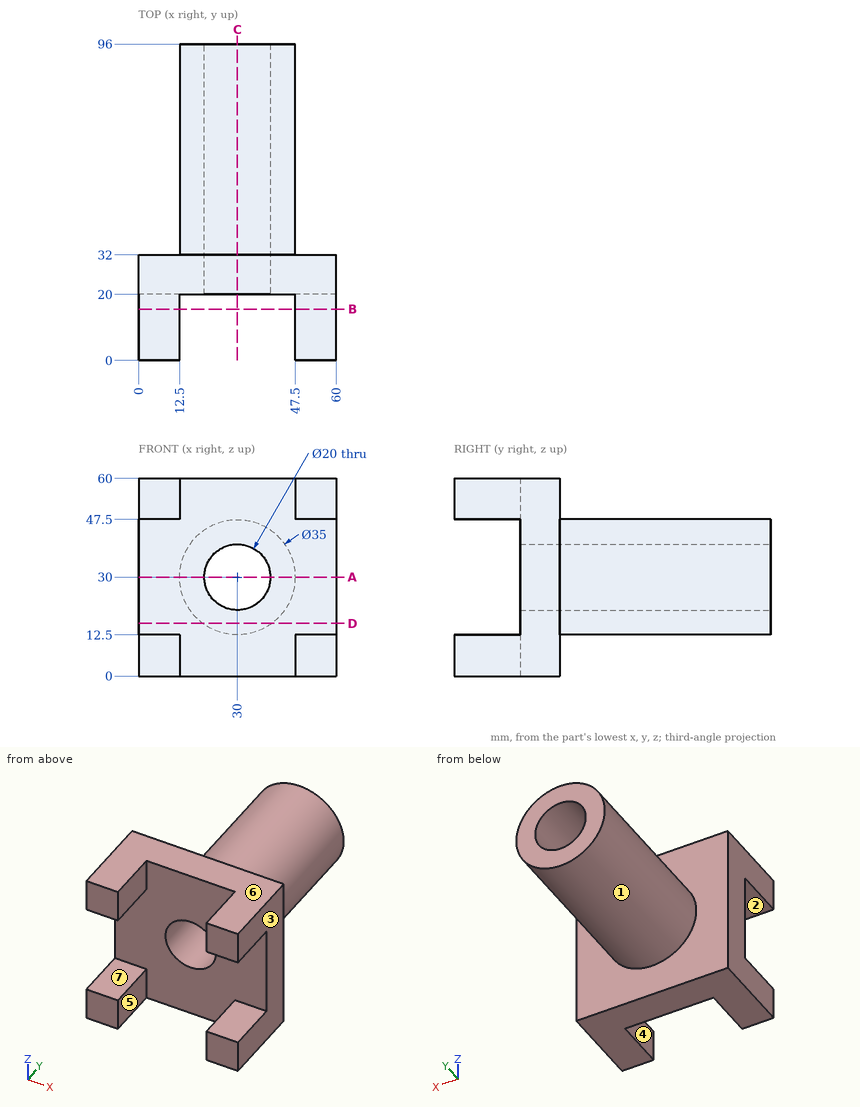
Geometry check sheet. Reference: drawing and pictorial views, mm from the part's lowest x, y, z. A direction names the side the tool comes from. Coordinates: 2 decimals unless noted, no trailing zeros. Write each loop counter-clockwise with the first axis right and the second up, starting at its lowest first coordinate (ties: lowest second). Pieces come first, ordered by that corner, then holes. Notation, with made-up numbers: M 46.25,-34 L 54.25,-34 A20 ccw 54.25,2 Z; hole C -36.75,3 d10. An arc over 180 degrees is marked long. Write item = value, one per line. Start each with the question number.
1. Sectioned sample at B-B (y = 15.5). Record the cut outline in (x, z), then the cut area to 3 significant figures.
2. Sectioned sample at D-D (z = 16). Record the cut outline in (x, y), then the cut area to 3 significant figures.
3. Sectioned sample at C-C (x = 30). Record the cut outline in (y, z).
4. Sectioned sample at A-A (z = 30). Record the cut outline in (x, y), then the cut area to 3 significant figures.
5. Tool access check on the marked faces 1, 2, 3 and 4. Record the directions out of +Z, -Z, +X, -X, +Y, -Y that give a thin tool (end or side, any length) a straight path to the whole face; none if there is none.
6. Thickness scan on probe 1 along Z at (x, y) = (30, 48.5); probe 2 along Y at (x, z) = (49.5, 49). Record the ranges inside material, lowest first.
7. Go/stop test with flat-tipped pins: pin 1 (8 mm diameter, centred on y = 73.5, z = 14, fed in from -X); pin 2 (4 mm diameter, centred on x = 16, z = 49, fed in from -Y); pin 3 (8 mm diameter, centred on y = 48, z = 11.5, fed in from -X). Record where each tip stops, or that it passes through.
8. Mould release check, pull along Z, two halves, no side actions. Record for the marked faces 5, 6 and 7: pulls with the +Z half, pulls with the -Z half, needs draft (parallel to the pull), parting line crosses it, or undercut.
The answers:
q1.outline = M 0,0 L 12.5,0 L 12.5,12.5 L 0,12.5 Z; M 0,47.5 L 12.5,47.5 L 12.5,60 L 0,60 Z; M 47.5,0 L 60,0 L 60,12.5 L 47.5,12.5 Z; M 47.5,47.5 L 60,47.5 L 60,60 L 47.5,60 Z
q1.area = 625 mm²
q2.outline = M 0,20 L 60,20 L 60,32 L 40.5,32 L 40.5,96 L 19.5,96 L 19.5,32 L 0,32 Z
q2.area = 2,060 mm²
q3.outline = M 20,0 L 32,0 L 32,12.5 L 96,12.5 L 96,20 L 20,20 Z; M 20,40 L 96,40 L 96,47.5 L 32,47.5 L 32,60 L 20,60 Z
q4.outline = M 0,20 L 20,20 L 20,96 L 12.5,96 L 12.5,32 L 0,32 Z; M 40,20 L 60,20 L 60,32 L 47.5,32 L 47.5,96 L 40,96 Z
q4.area = 1,440 mm²
q5.face_1 = +Y
q5.face_2 = +X, -X, -Y
q5.face_3 = +Z, -Z, +X, +Y, -Y
q5.face_4 = +Z, -Z, -Y
q6.probe_1 = 12.5 to 20, 40 to 47.5
q6.probe_2 = 0 to 32
q7.pin_1 = 17.26
q7.pin_2 = 20
q7.pin_3 = 20.2
q8.face_5 = needs draft
q8.face_6 = pulls with the +Z half
q8.face_7 = undercut
